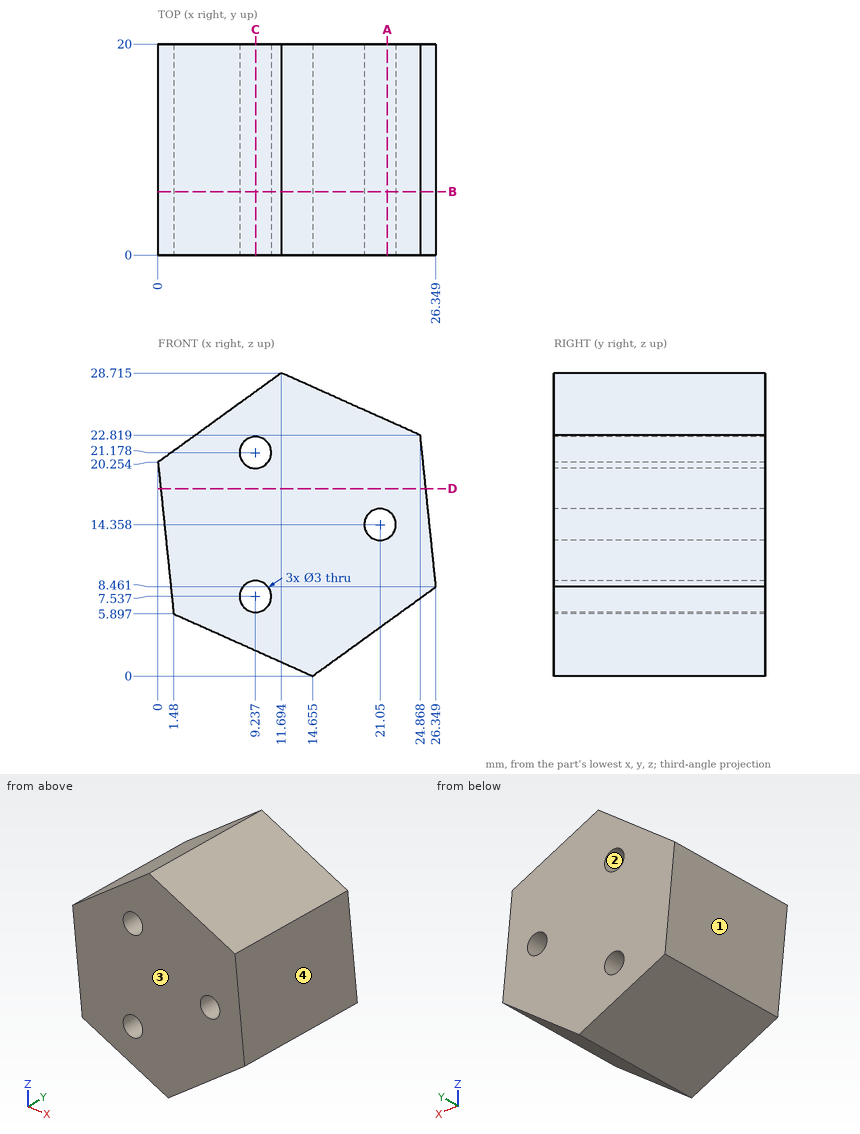
The drawing under review shows one solid part. Ordinate dimensions are in mm from its lowest x, y, z. Give positions to 0.01 mm unless a question says otherwise; leave off trailing zeros. Order: outer loops, then holes, each group sorted by start corner. A loop starts at its lowest first (then second) coordinate and runs counter-clockwise, first axis right, second up. Notation, with made-up numbers: (-26.75, 35.25) -> (22.25, 35.25) arc R10 cw to (22.25, 42.25) -> close; hole circle Ø7 at (22.25, 51). An arc over 180 degrees is marked (long way). Write item = value, one per line. Start each with the question number.
(1) We need section B-B on y = 6. State how many separate pieces and enclosed holes the cut face has, plus the area to 3 significant figures.
(2) We need section C-C on x = 9.25. Write out the cut boundary in (y, z).
(3) To check wall thickness, follow line 1 along Z through (x, y) = (8.5, 11.5) (1 decimal); line 2 along Z through (x, y) = (10, 10) (1 decimal); line 3 along X through (y, z) = (1.25, 7) (1 decimal). State the ranges of each line that lie inside material, in increasing order.
(4) We need section D-D on z = 17.75. Write out the cut boundary in (x, y), plus the area to 3 significant figures.
(5) We need section A-A on x = 21.75. Write out the cut boundary in (y, z) (1 decimal).
(6) For pin 1 (8 mm diameter, centred on y = 3.5, z = 22, fed in from +X) (1 decimal); pin 2 (2 mm diameter, centred on x = 3, y = 9.5, fed in from +Z); pin 3 (1 mm diameter, centred on x = 10, y = 13, fed in from -Z), all flat-tipped, find the tip position at first contact; note any pin that passes through.
(7) Mouldability with a two-part tool opening along X and no side actions: class the marked faces 1, 2, 3 and 4 as +X half, -X half, draft (parallel to the pull), parting line (faces both ways), or undercut.
Numbers:
q1.separate_pieces = 1
q1.enclosed_holes = 3
q1.area = 520 mm^2
q2.outline = (0, 2.42) -> (20, 2.42) -> (20, 6.04) -> (0, 6.04) -> close; (0, 9.04) -> (20, 9.04) -> (20, 19.68) -> (0, 19.68) -> close; (0, 22.68) -> (20, 22.68) -> (20, 26.95) -> (0, 26.95) -> close
q3.line_1 = 2.8 to 6.2, 8.8 to 19.9, 22.5 to 26.4
q3.line_2 = 2.1 to 6.2, 8.8 to 19.9, 22.5 to 27.5
q3.line_3 = 1.4 to 7.8, 10.6 to 24.3
q4.outline = (0.26, 0) -> (25.39, 0) -> (25.39, 20) -> (0.26, 20) -> close
q4.area = 503 mm^2
q5.outline = (0, 5.1) -> (20, 5.1) -> (20, 13) -> (0, 13) -> close; (0, 15.7) -> (20, 15.7) -> (20, 24.2) -> (0, 24.2) -> close
q6.pin_1 = 25.4
q6.pin_2 = 23.15
q6.pin_3 = 1.86
q7.face_1 = -X half
q7.face_2 = undercut
q7.face_3 = draft
q7.face_4 = +X half
